Geometry: final body of the model. Coordinates: model frame, mm. Face numbers are marked on the shaded views. Round coordinates to 2 decimals unless told otherwise and drop trailing zeros. Order: outer loops, then holes, each group sorted by start corner. A loop starts at its lowest first (then second) coordinate and runs counter-clockwise, first axis right, second up. Notation, with made-up numbers: M -29,72 L -13,72 A37 cw -13,109 Z; hole C 36,36 d3. An arc over 180 degrees is marked long. Return JSON: item names as keys, results as strings. Group by question number.
Q1. Cut plane C-C on z = 174.5. Output: boundary loops of the cut face in (x, y), and give its area (3 significant figures).
Q2. Cut plane B-B on y = 0. Output: boundary loops of the cut face in (x, z).
Q3. Mould query, pull axis Y, two halves, no side actions, for the marked faces 1, 2 and 3. Classes: released by +Y, released by -Y, zero draft, split by the parting line, or undercut.
Q4. Contact query for a flat-ended pin moving along its axis: pin 1 (12 mm diameter, centred on x = -157, z = 73, fed in from -Y). Output: stop coordinate, or through.
Q5. Cut plane D-D on z = -35. Output: boundary loops of the cut face in (x, y).
Q6. Ray query, probe 1 along Y at (x, z) = (0, 112); probe 2 along Y at (x, z) = (-477, 191); probe 3 along X at (y, z) = (-584, 132). Return the intervals inside material, ascending.
Q7. Cut plane A-A on x = 0. Output: boundary loops of the cut face in (y, z).
```python
from build123d import *

# Parameters (mm, degrees)
F0_W     = 990.6
F0_H     = 1905
F1_DEPTH = 254
F2_W     = 50.8
F2_H     = 50.8
F3_DEPTH = 330.2
F6_R     = 178.695412
F7_DEPTH = 584.201
F8_R     = 54.530452
F9_DEPTH = 25.4


with BuildPart() as f1:
    # F0 (on Top) → F1 (new body)
    with BuildSketch(Plane.XY):
        Rectangle(F0_W, F0_H)
    extrude(amount=F1_DEPTH)

    # F2 (on face) → F3 (join)
    with BuildSketch(Plane(origin=(0, 0, 0), x_dir=(1, 0, 0), z_dir=(0, 0, -1))):
        with Locations((-469.9, 927.1)):
            Rectangle(F2_W, F2_H)
    extrude(amount=F3_DEPTH)

    # F4: F1 across plane


with BuildPart() as f1_1:
    add(f1.part)
    add(f1.part.mirror(Plane.YZ))

    # F5: F1 across plane


with BuildPart() as f1_2:
    add(f1_1.part)
    add(f1_1.part.mirror(Plane.XZ))

    # F6 (on face) → F7 (cut, through all)
    with BuildSketch(Plane.XY.offset(254)):
        Circle(F6_R)
    extrude(amount=-F7_DEPTH, mode=Mode.SUBTRACT)

    # F8 (on face) → F9 (join)
    with BuildSketch(Plane(origin=(0, 0, -330.2), x_dir=(1, 0, 0), z_dir=(0, 0, -1))):
        with Locations((-480.838805, 929.906964)):
            Circle(F8_R)
    extrude(amount=-F9_DEPTH)


solid = f1_2.part
```
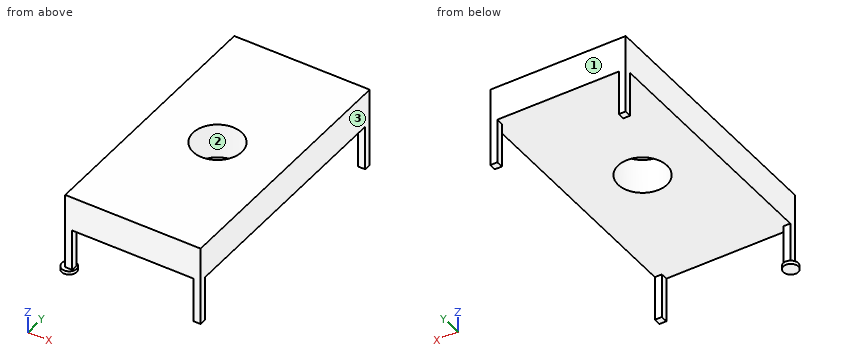
Result sheet:
{
 "1": {"outline": "M -495.3,-952.5 L 495.3,-952.5 L 495.3,952.5 L -495.3,952.5 Z; hole C 0,0 d357.39", "area": "1,790,000 mm²"},
 "2": {"outline": "M -495.3,0 L -178.7,0 L -178.7,254 L -495.3,254 Z; M 178.7,0 L 495.3,0 L 495.3,254 L 178.7,254 Z"},
 "3": {"face 1": "released by +Y", "face 2": "undercut", "face 3": "zero draft"},
 "4": {"pin 1": "stops at y = -952.5"},
 "5": {"outline": "M -495.3,-952.5 L -444.5,-952.5 L -444.5,-901.7 L -495.3,-901.7 Z; M -495.3,901.7 L -444.5,901.7 L -444.5,952.5 L -495.3,952.5 Z; M 444.5,-952.5 L 495.3,-952.5 L 495.3,-901.7 L 444.5,-901.7 Z; M 444.5,901.7 L 495.3,901.7 L 495.3,952.5 L 444.5,952.5 Z"},
 "6": {"probe 1": "y = -952.5 to -178.7, 178.7 to 952.5", "probe 2": "y = -952.5 to 952.5", "probe 3": "x = -495.3 to 495.3"},
 "7": {"outline": "M -952.5,0 L -178.7,0 L -178.7,254 L -952.5,254 Z; M 178.7,0 L 952.5,0 L 952.5,254 L 178.7,254 Z"}
}
